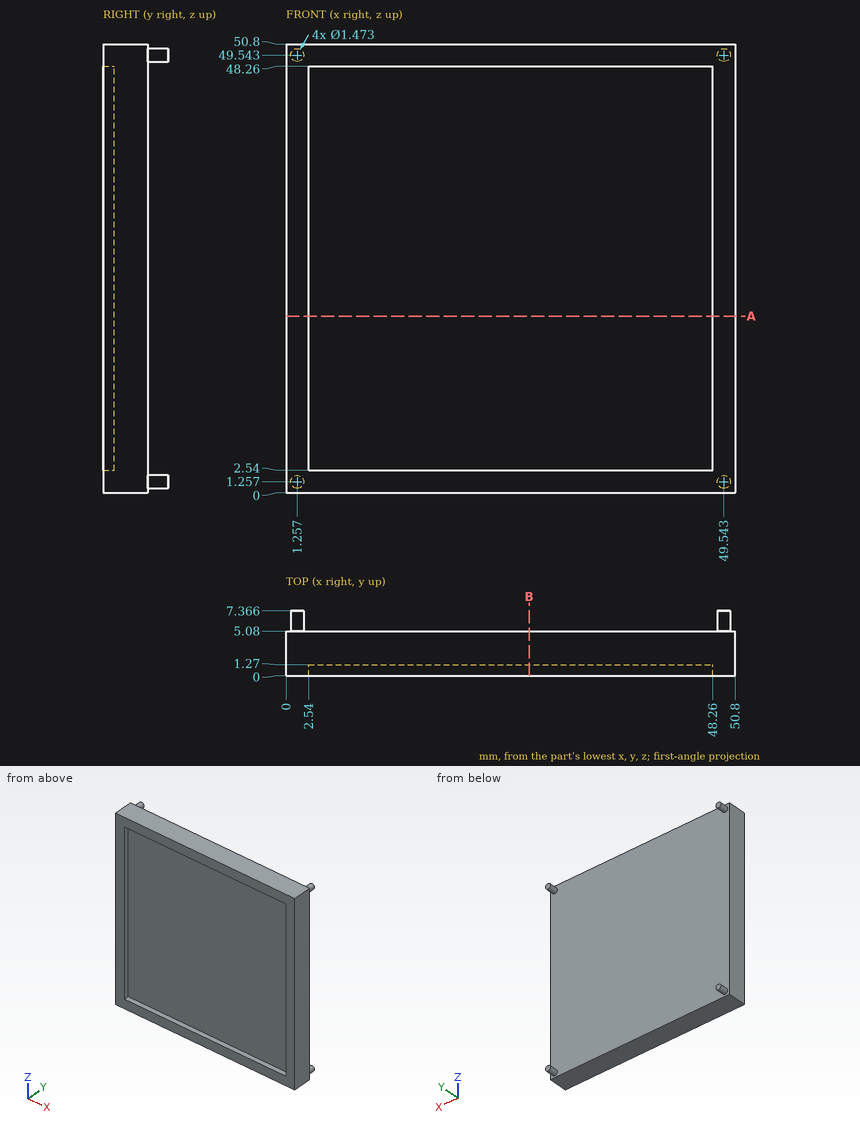
The drawing under review shows one solid part. Ordinate dimensions are in mm from its lowest x, y, z. Give positions to 0.01 mm unless a question says otherwise; leave off trailing zeros. Loops run counter-clockwise (first coordinate to the right, second up) from the corner with the lowest first, then second, coordinate; pieces in that order, holes last. Notation, with made-up numbers: M -3.75,72.25 L 17.25,72.25 A26 cw 17.25,93.25 Z; hole C 58.25,45 d4. An arc over 180 degrees is marked long. One line per item, written item: value. Start each with the question number.
Q1. For L1, parallel to X at y = 1, z = 25; L2, parallel to Y at x = 21, z = 17, list the stretches that pass through material, from the lowest coordinate up.
Q2. Add section A-A (z = 20). Give the boundary of the cut face in (x, y), and give its area (3 significant figures).
Q3. Add section B-B (x = 27.5). Give the boundary of the cut face in (y, z), and give its area (3 significant figures).
Q4. Clearance check with flat-ended pins moving along their axes: pin 1 Ø5 at (x, z) = (23.5, 14.5) entering from +Y; pin 2 Ø2 at (x, z) = (34.5, 41.5) entering from -Y. State where each tip first meets the part, or that it passes through.
Reply:
1. L1: 0 to 2.54, 48.26 to 50.8
1. L2: 1.27 to 5.08
2. outline: M 0,0 L 2.54,0 L 2.54,1.27 L 48.26,1.27 L 48.26,0 L 50.8,0 L 50.8,5.08 L 0,5.08 Z
2. area: 200 mm²
3. outline: M 0,0 L 5.08,0 L 5.08,50.8 L 0,50.8 L 0,48.26 L 1.27,48.26 L 1.27,2.54 L 0,2.54 Z
3. area: 200 mm²
4. pin 1: y = 5.08
4. pin 2: y = 1.27
